from build123d import *

# Parameters (mm, degrees)
BOSS_EXTRUDE1_DEPTH = 150
CUT_EXTRUDE7_START  = -7.5
SKETCH2_R           = 9
CUT_EXTRUDE7_DEPTH  = 135
CIRPATTERN1_COUNT   = 6
SKETCH3_R           = 19.05
CUT_EXTRUDE8_DEPTH  = 159.205648445
CUT_EXTRUDE9_START  = -5.9
SKETCH5_R           = 35.56
CUT_EXTRUDE9_DEPTH  = 5.9
SKETCH6_R           = 30.56
BOSS_EXTRUDE2_DEPTH = 5
SKETCH7_R           = 35.56
BOSS_EXTRUDE3_DEPTH = 2.5


with BuildPart() as part:
    # Sketch1 → Boss-Extrude1 (new body)
    with BuildSketch(Plane(origin=(0, 0, 0), x_dir=(1, 0, 0), z_dir=(0, 1, 0))):
        with BuildLine():
            ThreePointArc((-35.56, 0), (0, 35.56), (35.56, 0))
            ThreePointArc((35.56, 0), (0, -35.56), (-35.56, 0))
        make_face()
    extrude(amount=BOSS_EXTRUDE1_DEPTH)

    # Sketch2 → Cut-Extrude7 (cut)
    with BuildSketch(Plane(origin=(0, 0, 0), x_dir=(-1, 0, 0), z_dir=(0, -1, 0)).offset(CUT_EXTRUDE7_START)):
        with Locations((0, 29)):
            Circle(SKETCH2_R)
    cut_extrude7 = extrude(amount=-CUT_EXTRUDE7_DEPTH, mode=Mode.SUBTRACT)

    # CirPattern1: Cut-Extrude7 ×6 about axis
    cirpattern1_axis = Axis((0, 0, 0), (0, 1, 0))
    for i in range(1, CIRPATTERN1_COUNT):
        add(cut_extrude7.rotate(cirpattern1_axis, i * 360 / CIRPATTERN1_COUNT), mode=Mode.SUBTRACT)

    # Sketch3 → Cut-Extrude8 (cut, through all)
    with BuildSketch(Plane(origin=(0, 0, 0), x_dir=(-1, 0, 0), z_dir=(0, -1, 0))):
        with Locations(Location((0, 0, 0), (0, 0, 90))):
            Circle(SKETCH3_R)
    extrude(amount=-CUT_EXTRUDE8_DEPTH, mode=Mode.SUBTRACT)

    # Sketch5 → Cut-Extrude9 (cut)
    with BuildSketch(Plane(origin=(0, 150, 0), x_dir=(1, 0, 0), z_dir=(0, 1, 0)).offset(CUT_EXTRUDE9_START)):
        with Locations(Location((0, 0, 0), (0, 0, 90))):
            Circle(SKETCH5_R)
    extrude(amount=CUT_EXTRUDE9_DEPTH, mode=Mode.SUBTRACT)

    # Sketch6 → Boss-Extrude2 (add)
    with BuildSketch(Plane(origin=(0, 144.1, 0), x_dir=(1, 0, 0), z_dir=(0, 1, 0))):
        with Locations(Location((0, 0, 0), (0, 0, 270))):
            Circle(SKETCH6_R)
    extrude(amount=BOSS_EXTRUDE2_DEPTH)

    # Sketch7 → Boss-Extrude3 (add)
    with BuildSketch(Plane(origin=(0, 149.1, 0), x_dir=(1, 0, 0), z_dir=(0, 1, 0))):
        with Locations(Location((0, 0, 0), (0, 0, 90))):
            Circle(SKETCH7_R)
    extrude(amount=BOSS_EXTRUDE3_DEPTH)


solid = part.part
Can you work these out from the model? Positions are in its coordinate system, mm. A direction names the side the tool comes from. Give positions to 0.01 mm unless a question says otherwise; leave off trailing zeros. Loops run counter-clockwise (first coordinate to the right, second up) from the corner with the lowest first, then second, coordinate; pieces in that order, holes last. Notation, with made-up numbers: (-20, -6) -> (26, -6) arc R21 ccw to (26, 15) -> close; hole circle Ø2 at (-33, -14). An arc over 180 degrees is marked (long way). Return JSON: item names as keys, results as strings.
Q1. For pin 1 Ø4 at (x, y) = (5.5, 112) entering from +Z; pin 2 Ø4 at (x, y) = (3, 68.5) entering from +Z; pin 3 Ø3 at (y, z) = (27, -5.5) entering from +X, each with a flat end and sliding along its axis, tell me the tip position at first contact or that it passes through.
Checks:
{"pin 1": "stops at z = 34.91", "pin 2": "stops at z = 21.52", "pin 3": "stops at x = 35.33"}
Q2. I want a section at A-A, the plane z = 0. List the corners of the cut face in (x, y) for me, then the cut area to 3 significant figures.
Checks:
{"outline": "(-35.56, 0) -> (-19.05, 0) -> (-19.05, 144.1) -> (19.05, 144.1) -> (19.05, 0) -> (35.56, 0) -> (35.56, 144.1) -> (30.56, 144.1) -> (30.56, 149.1) -> (35.56, 149.1) -> (35.56, 151.6) -> (-35.56, 151.6) -> (-35.56, 149.1) -> (-30.56, 149.1) -> (-30.56, 144.1) -> (-35.56, 144.1) -> close", "area": "5,240 mm2"}
Q3. I want a section at D-D, the plane x = 14. List the corners of the cut face in (y, z) for me, then the cut area to 3 significant figures.
Checks:
{"outline": "(0, -32.69) -> (144.1, -32.69) -> (144.1, -27.16) -> (149.1, -27.16) -> (149.1, -32.69) -> (151.6, -32.69) -> (151.6, 32.69) -> (149.1, 32.69) -> (149.1, 27.16) -> (144.1, 27.16) -> (144.1, 32.69) -> (0, 32.69) -> (0, 12.92) -> (144.1, 12.92) -> (144.1, -12.92) -> (0, -12.92) -> close", "area": "6,130 mm2"}
Q4. On a 3-axis mill with a long thin cutter (end or side, diameter ignored), from which of +Z, -Z, +X, -X, +Y, -Y can I reach the whole of each face in a straight line? I mean faces 1 (the face through (-17.18, 74.05, -10.25)), 2 (the face through (-11.59, 71.04, 15.12)), 3 (the face through (33.92, 71.04, 10.68)). Say none if no direction works.
Checks:
{"face 1": "none", "face 2": "-Y", "face 3": "+Y, -Y"}
Q5. We'd pull the mould along Z, two halves only. Please class faces 4 (the face through (17.47, 74.05, -9.75)), 5 (the face through (-15, 0, 15)), 6 (the face through (-11.7, 146.56, 28.23)): released by +Z, released by -Z, zero draft, split by the parting line, or undercut.
Checks:
{"face 4": "undercut", "face 5": "zero draft", "face 6": "split by the parting line"}
Q6. I want a section at B-B, the plane y = 73. List the corners of the cut face in (x, z) for me.
Checks:
{"outline": "(-33.62, -11.57) arc R9 cw (long way) to (-26.83, -23.33) arc R35.56 ccw to (-6.79, -34.91) arc R9 cw (long way) to (6.79, -34.91) arc R35.56 ccw to (26.83, -23.33) arc R9 cw (long way) to (33.62, -11.57) arc R35.56 ccw to (33.62, 11.57) arc R9 cw (long way) to (26.83, 23.33) arc R35.56 ccw to (6.79, 34.91) arc R9 cw (long way) to (-6.79, 34.91) arc R35.56 ccw to (-26.83, 23.33) arc R9 cw (long way) to (-33.62, 11.57) arc R35.56 ccw to start; hole circle Ø38.1 at (0, 0)"}
Q7. I want a section at C-C, the plane x = -21. List the corners of the cut face in (y, z) for me.
Checks:
{"outline": "(0, -28.7) -> (144.1, -28.7) -> (144.1, -22.2) -> (149.1, -22.2) -> (149.1, -28.7) -> (151.6, -28.7) -> (151.6, 28.7) -> (149.1, 28.7) -> (149.1, 22.2) -> (144.1, 22.2) -> (144.1, 28.7) -> (0, 28.7) -> close; hole (7.5, -22.5) -> (142.5, -22.5) -> (142.5, -6.5) -> (7.5, -6.5) -> close; hole (7.5, 6.5) -> (142.5, 6.5) -> (142.5, 22.5) -> (7.5, 22.5) -> close"}
Q8. I need wall thicknesses on probe 1 along Y at (x, z) = (-28, 13); probe 2 along Z at (x, y) = (25, 20); probe 3 along Z at (x, y) = (25.5, 57). Which ranges of each line are inside material? Lowest first, please.
Checks:
{"probe 1": "y = 0 to 7.5, 142.5 to 144.1, 149.1 to 151.6", "probe 2": "z = -25.29 to -23.5, -5.5 to 5.5, 23.5 to 25.29", "probe 3": "z = -24.78 to -23.49, -5.51 to 5.51, 23.49 to 24.78"}
